Part model, mm, in its own coordinate system. Face numbers are marked on the shaded views. A direction names the side the tool comes from. Round coordinates to 2 decimals unless told otherwise and drop trailing zeros. Order: outer loops, then holes, each group sorted by start corner. A loop starts at its lowest first (then second) coordinate and runs counter-clockwise, first axis right, second up. Notation, with made-up numbers: (-2.5, -0.5) - (40.5, -0.5) arc R19 ccw to (40.5, 33.5) - close; hole circle Ø5 at (-35, 25). An arc over 180 degrees is marked (long way). Return JSON: item names as keys, results as strings. Group by question number.
Item 1: Probe probe 1 along Y at (x, z) = (-1, -2.5); probe 2 along Z at (x, y) = (-1.5, -9); probe 3 along Y at (x, z) = (1, 0.25) (3 decimals). List the from-to ranges inside material, lowest first.
Item 2: Saw through at A-A on y = 0.75. List the corners of the cut face in (x, z).
Item 3: Tool access for the marked faces 1 and 2: list every direction of +Z, -Z, +X, -X, +Y, -Y with a clear straight run to the whole face (end or side of a thin tool).
Item 4: Drop flat-ended pins along their axis: pin 1 (1 mm diameter, centred on y = -10.5, z = -1.5, fed in from +X); pin 2 (1.5 mm diameter, centred on x = 0.5, y = -5.5, fed in from +Z); pin 3 (1 mm diameter, centred on x = 1, z = -0.5, fed in from +Y). Give the stop position or say it passes through.
Item 5: Two-plate mould, pull along X, no slides. Class the marked faces 3, 4 and 5: released by +X, released by -X, zero draft, split by the parting line, or undercut.
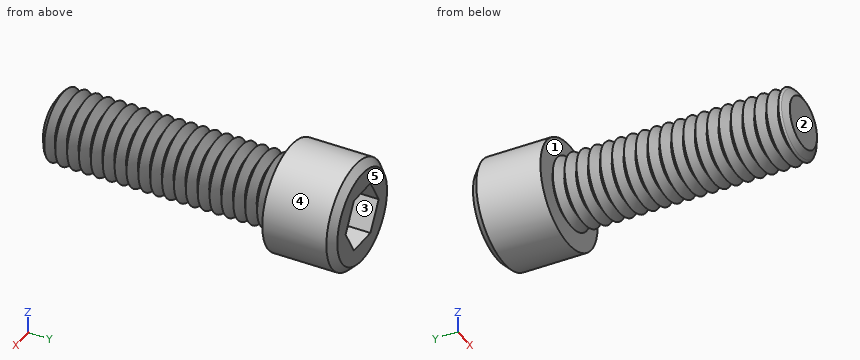
```python
from build123d import *

# Parameters (mm, degrees)
HEX_CUT_DRIVEN_DEPTH = 3.3782


with BuildPart() as part:
    # Sketch3 → Shank Revolve ( driven ) (revolve)
    with BuildSketch(Plane.XY, mode=Mode.PRIVATE) as shank_revolve_driven_sk:
        Polygon((0, 1.4478), (0, -15.875), (1.9304, -15.875), (2.413, -15.3924), (2.413, 1.4478), align=None)
    revolve(shank_revolve_driven_sk.sketch.rotate(Axis((0, -50, 0), (0, 1, 0)), 90), axis=Axis((0, -50, 0), (0, 1, 0)))

    # Sketch4 → Thread Revolve Cut ( driven ) (revolve, cut)
    with BuildSketch(Plane.XY, mode=Mode.PRIVATE) as thread_revolve_cut_driven_sk:
        Polygon((1.7164269, 3.429), (2.413, 3.831166667), (3.217333333, 3.831166667), (3.217333333, -17.885833333), (2.413, -17.885833333), (1.7164269, -17.483666667), (2.413, -17.0815), (1.7164269, -16.679333333), (2.413, -16.277166667), (1.7164269, -15.875), (2.413, -15.472833333), (1.7164269, -15.070666667), (2.413, -14.6685), (1.7164269, -14.266333333), (2.413, -13.864166667), (1.7164269, -13.462), (2.413, -13.059833333), (1.7164269, -12.657666667), (2.413, -12.2555), (1.7164269, -11.853333333), (2.413, -11.451166667), (1.7164269, -11.049), (2.413, -10.646833333), (1.7164269, -10.244666667), (2.413, -9.8425), (1.7164269, -9.440333333), (2.413, -9.038166667), (1.7164269, -8.636), (2.413, -8.233833333), (1.7164269, -7.831666667), (2.413, -7.4295), (1.7164269, -7.027333333), (2.413, -6.625166667), (1.7164269, -6.223), (2.413, -5.820833333), (1.7164269, -5.418666667), (2.413, -5.0165), (1.7164269, -4.614333333), (2.413, -4.212166667), (1.7164269, -3.81), (2.413, -3.407833333), (1.7164269, -3.005666667), (2.413, -2.6035), (1.7164269, -2.201333333), (2.413, -1.799166667), (1.7164269, -1.397), (2.413, -0.994833333), (1.7164269, -0.592666667), (2.413, -0.1905), (1.7164269, 0.211666667), (2.413, 0.613833333), (1.7164269, 1.016), (2.413, 1.418166667), (1.7164269, 1.820333333), (2.413, 2.2225), (1.7164269, 2.624666667), (2.413, 3.026833333), align=None)
    revolve(thread_revolve_cut_driven_sk.sketch.rotate(Axis((0, -50, 0), (0, 1, 0)), 90), axis=Axis((0, -50, 0), (0, 1, 0)), mode=Mode.SUBTRACT)

    # Sketch5 → Head Revolve ( driven ) (revolve)
    with BuildSketch(Plane.XY, mode=Mode.PRIVATE) as head_revolve_driven_sk:
        Polygon((0, 4.826), (0, 0), (3.6195, 0), (3.6195, 4.3434), (3.1369, 4.826), align=None)
    revolve(head_revolve_driven_sk.sketch.rotate(Axis((0, -50, 0), (0, 1, 0)), 90), axis=Axis((0, -50, 0), (0, 1, 0)))

    # Sketch2 → Hex Cut ( driven ) (cut)
    with BuildSketch(Plane(origin=(0, 4.826, 0), x_dir=(-1, 0, 0), z_dir=(0, 1, 0))):
        Polygon((-2.089719299, 0), (-1.04485965, -1.80975), (1.04485965, -1.80975), (2.089719299, 0), (1.04485965, 1.80975), (-1.04485965, 1.80975), align=None)
    extrude(amount=-HEX_CUT_DRIVEN_DEPTH, mode=Mode.SUBTRACT)


solid = part.part
```
Filled in:
{
 "1": {"probe 1": "y = 0 to 4.83", "probe 2": "z = -1.8 to 1.8", "probe 3": "y = -15.875 to 1.448"},
 "2": {"outline": "circle Ø7.24 at (0, 0)"},
 "3": {"face 1": "none", "face 2": "+Z, -Z, +X, -X, -Y"},
 "4": {"pin 1": "stops at x = 2.19", "pin 2": "stops at z = 2.41", "pin 3": "stops at y = 1.45"},
 "5": {"face 3": "undercut", "face 4": "split by the parting line", "face 5": "zero draft"}
}
